Build history of the part. All positions in model axes, mm. Face numbers are marked on the shaded views. A direction names the side the tool comes from. Round coordinates to 2 decimals unless told otherwise and drop trailing zeros. Write each loop counter-clockwise with the first axis right and the second up, starting at its lowest first coordinate (ties: lowest second). Pieces come first, ordered by that corner, then holes. Notation, with made-up numbers: (57, 23) - (65, 23) arc R22 cw to (65, 62) - close; hole circle Ø2 at (-11.5, 48.25). An arc over 180 degrees is marked (long way). One line per question, with ' | ' between items.
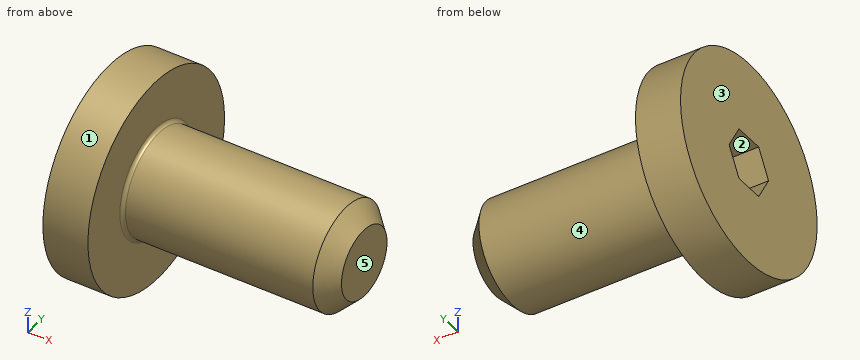
from build123d import *

# Parameters (mm, degrees)
CUT_EXTRUDE1_DEPTH = 2


with BuildPart() as part:
    # Sketch1 → Revolve1 (revolve)
    with BuildSketch(Plane.XY, mode=Mode.PRIVATE) as revolve1_sk:
        with BuildLine():
            Line((-1.3, 0), (6, 0))
            Line((6, 0), (6, -1))
            Line((6, -1), (5.5, -1.5))
            Line((5.5, -1.5), (0.1, -1.5))
            ThreePointArc((0.1, -1.5), (0.029289322, -1.529289322), (0, -1.6))
            Line((0, -1.6), (0, -3))
            Line((0, -3), (-1.3, -3))
            Line((-1.3, -3), (-1.3, 0))
        make_face()
    revolve(revolve1_sk.sketch.rotate(Axis((6, 0, 0), (-1, 0, 0)), 180), axis=Axis((6, 0, 0), (-1, 0, 0)))

    # Sketch2 → Cut-Extrude1 (cut)
    with BuildSketch(Plane.ZY.offset(1.3)):
        Polygon((0, 0.866025404), (-0.75, 0.433012702), (-0.75, -0.433012702), (0, -0.866025404), (0.75, -0.433012702), (0.75, 0.433012702), align=None)
    extrude(amount=-CUT_EXTRUDE1_DEPTH, mode=Mode.SUBTRACT)


solid = part.part
Q1. Drop a flat-ended pin along its axis: pin 1 (1.5 mm diameter, centred on x = 4.5, y = 1, fed in from -Z). Give the stop position or say it passes through.
Found:
pin 1: z = -1.48
Q2. Drill centre lines: L1, parallel to X at y = -1.3, z = 2.4; L2, parallel to X at y = 0.35, z = -0.55; L3, parallel to Z at x = 1, y = -0.5. Where is each one in solid material? Low to high. Write a range as from..to.
Found:
L1: -1.3..0 | L2: 0.7..6 | L3: -1.41..1.41
Q3. Saw through at C-C, the plane x = 5.75. List the corners of the cut face in (y, z), then the cut area to 3 significant figures.
Found:
outline: circle Ø2.5 at (0, 0) | area: 4.91 mm^2
Q4. Saw through at D-D, the plane z = -1.7. List the corners of the cut face in (x, y), then the cut area to 3 significant figures.
Found:
outline: (-1.3, -2.47) - (0, -2.47) - (0, 2.47) - (-1.3, 2.47) - close | area: 6.43 mm^2
Q5. Saw through at A-A, the plane y = 0. List the corners of the cut face in (x, z).
Found:
outline: (-1.3, -3) - (0, -3) - (0, -1.6) arc R0.1 cw to (0.1, -1.5) - (5.5, -1.5) - (6, -1) - (6, 1) - (5.5, 1.5) - (0.1, 1.5) arc R0.1 cw to (0, 1.6) - (0, 3) - (-1.3, 3) - (-1.3, 0.75) - (0.7, 0.75) - (0.7, -0.75) - (-1.3, -0.75) - close
Q6. Saw through at B-B, the plane x = 0.5. List the corners of the cut face in (y, z).
Found:
outline: circle Ø3 at (0, 0); hole (-0.87, 0) - (-0.43, -0.75) - (0.43, -0.75) - (0.87, 0) - (0.43, 0.75) - (-0.43, 0.75) - close
Q7. Which spindle directions (+Z, -Z, +X, -X, +Y, -Y) get a long thin tool onto all of the face, cutting with end or side? Do the marked faces 4 and 5. Say none if no direction does.
Found:
face 4: +X | face 5: +Z, -Z, +X, +Y, -Y
Q8. Pull direction Y, two halves, no side cores. Call the marked faces 1, 2 and 3: +Y half, -Y half, draft (parallel to the pull), parting line (faces both ways), or undercut.
Found:
face 1: parting line | face 2: undercut | face 3: draft
